Geometry check sheet. Reference: the model listing, model coordinates, mm. A direction names the side the tool comes from. Give positions to 0.01 mm unless a question says otherwise; leave off trailing zeros. Loops run counter-clockwise (first coordinate to the right, second up) from the corner with the lowest first, then second, coordinate; pieces in that order, holes last. Notation, with made-up numbers: (86.5, 65) -> (112.5, 65) arc R16 cw to (112.5, 81) -> close; hole circle Ø6 at (40.5, 42). An arc over 180 degrees is marked (long way). Answer in a Markdown table with one row per item. Add a question column.
```python
from build123d import *

# Parameters (mm, degrees)
SKETCH1_W           = 99
SKETCH1_H           = 54.5
SKETCH1_R           = 1.6
SKETCH1_W_2         = 14.25
SKETCH1_H_2         = 14.25
BOSS_EXTRUDE1_DEPTH = 2
FILLET1_R           = 1.5


with BuildPart() as part:
    # Sketch1 → Boss-Extrude1 (new body)
    with BuildSketch(Plane(origin=(0, 0, 0), x_dir=(1, 0, 0), z_dir=(0, 1, 0))):
        Rectangle(SKETCH1_W, SKETCH1_H)
        with Locations(Location((-45.5, 23.25, 0), (0, 0, 270))):
            Circle(SKETCH1_R, mode=Mode.SUBTRACT)
        with Locations(Location((45.5, 23.25, 0), (0, 0, 90))):
            Circle(SKETCH1_R, mode=Mode.SUBTRACT)
        with Locations(Location((45.5, -23.25, 0), (0, 0, 270))):
            Circle(SKETCH1_R, mode=Mode.SUBTRACT)
        with Locations(Location((-45.5, -23.25, 0), (0, 0, 90))):
            Circle(SKETCH1_R, mode=Mode.SUBTRACT)
        with Locations((-33.375, 11.125)):
            Rectangle(SKETCH1_W_2, SKETCH1_H_2, mode=Mode.SUBTRACT)
        with Locations((-11.125, 11.125)):
            Rectangle(SKETCH1_W_2, SKETCH1_H_2, mode=Mode.SUBTRACT)
        with Locations((11.125, 11.125)):
            Rectangle(SKETCH1_W_2, SKETCH1_H_2, mode=Mode.SUBTRACT)
        with Locations((33.375, 11.125)):
            Rectangle(SKETCH1_W_2, SKETCH1_H_2, mode=Mode.SUBTRACT)
        with Locations((33.375, -11.125)):
            Rectangle(SKETCH1_W_2, SKETCH1_H_2, mode=Mode.SUBTRACT)
        with Locations((11.125, -11.125)):
            Rectangle(SKETCH1_W_2, SKETCH1_H_2, mode=Mode.SUBTRACT)
        with Locations((-11.125, -11.125)):
            Rectangle(SKETCH1_W_2, SKETCH1_H_2, mode=Mode.SUBTRACT)
        with Locations((-33.375, -11.125)):
            Rectangle(SKETCH1_W_2, SKETCH1_H_2, mode=Mode.SUBTRACT)
    extrude(amount=BOSS_EXTRUDE1_DEPTH)

    # Fillet1
    fillet1_edges = [part.edges().sort_by_distance(p)[0] for p in [
        (-45.5, 2, -24.85),
        (45.5, 2, -21.65),
        (45.5, 2, 21.65),
        (-45.5, 2, 24.85),
    ]]
    fillet(fillet1_edges, radius=FILLET1_R)


solid = part.part
```
1. Material ranges on L1, parallel to X at y = 0.75, z = 6.5; L2, parallel to Z at x = -15, y = 0.8; L3, parallel to X at y = 0.35, z = 23.25, recorded low to high. Write a range as from..to.
2. Sectioned sample at C-C (z = -23.25). Enter the section's corners in (x, y), plus the area to 3 significant figures.
3. Sectioned sample at A-A (x = 38). Enter the section's corners in (y, z).
4. Gauge pin test, flat end, axial feed: pin 1 Ø1 at (x, z) = (-38.5, -13.5) entering from +Y. Record the tip position at first contact, or that the pin passes through.
5. Sectioned sample at B-B (z = 14.5). Enter the section's corners in (x, y), plus the area to 3 significant figures.
6. Access from +Z, -Z, +X, -X, +Y, -Y to the whole of each face (thin tool, end or side, straight path). Record for faces 4 (the face through (-33, 1, 4)), 5 (the face through (-49.5, 1, 0)).
7. Release check for a two-part mould opening along X. For faces 1 (the face through (-1, 1, -27.25)), 2 (the face through (49.5, 1, 0)), 3 (the face through (33, 1, 18.25)) record: released by +X, released by -X, zero draft, split by the parting line, or undercut.
Response:
| question | item | result |
|---|---|---|
| 1 | L1 | x = -49.5..-40.5, -26.25..-18.25, -4..4, 18.25..26.25, 40.5..49.5 |
| 1 | L2 | z = -27.25..-18.25, -4..4, 18.25..27.25 |
| 1 | L3 | x = -49.5..-47.1, -43.9..43.9, 47.1..49.5 |
| 2 | outline | (-49.5, 0) -> (-47.1, 0) -> (-47.1, 0.5) arc R1.5 ccw to (-48.6, 2) -> (-49.5, 2) -> close; (-43.9, 0) -> (43.9, 0) -> (43.9, 0.5) arc R1.5 ccw to (42.4, 2) -> (-42.4, 2) arc R1.5 ccw to (-43.9, 0.5) -> close; (47.1, 0) -> (49.5, 0) -> (49.5, 2) -> (48.6, 2) arc R1.5 ccw to (47.1, 0.5) -> close |
| 2 | area | 183 mm2 |
| 3 | outline | (0, -27.25) -> (2, -27.25) -> (2, -18.25) -> (0, -18.25) -> close; (0, -4) -> (2, -4) -> (2, 4) -> (0, 4) -> close; (0, 18.25) -> (2, 18.25) -> (2, 27.25) -> (0, 27.25) -> close |
| 4 | pin 1 | passes through |
| 5 | outline | (-49.5, 0) -> (-40.5, 0) -> (-40.5, 2) -> (-49.5, 2) -> close; (-26.25, 0) -> (-18.25, 0) -> (-18.25, 2) -> (-26.25, 2) -> close; (-4, 0) -> (4, 0) -> (4, 2) -> (-4, 2) -> close; (18.25, 0) -> (26.25, 0) -> (26.25, 2) -> (18.25, 2) -> close; (40.5, 0) -> (49.5, 0) -> (49.5, 2) -> (40.5, 2) -> close |
| 5 | area | 84.0 mm2 |
| 6 | face 4 | +Y, -Y |
| 6 | face 5 | +Z, -Z, -X, +Y, -Y |
| 7 | face 1 | zero draft |
| 7 | face 2 | released by +X |
| 7 | face 3 | undercut |
